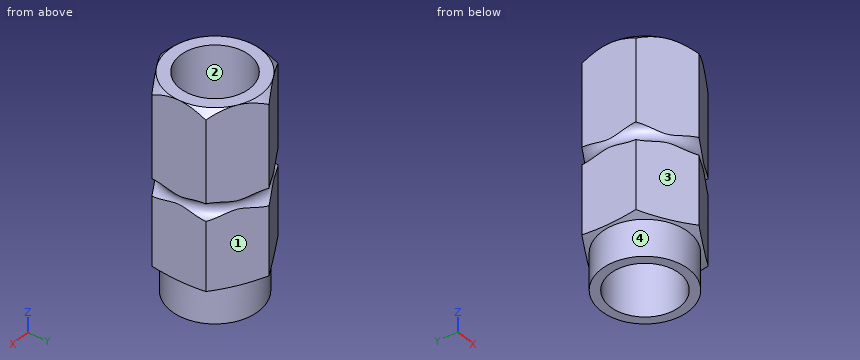
```python
from build123d import *

# Parameters (mm, degrees)
SKETCH1_R      = 9.525
EXTRUDE1_DEPTH = 59
SKETCH2_R      = 2.38125


with BuildPart() as part:
    # Sketch1 → Extrude1 (new body)
    with BuildSketch(Plane.XY):
        Polygon((-12.7, 7.332348419), (-12.7, -7.332348419), (0, -14.664696837), (12.7, -7.332348419), (12.7, 7.332348419), (0, 14.664696837), align=None)
        Circle(SKETCH1_R, mode=Mode.SUBTRACT)
    extrude(amount=-EXTRUDE1_DEPTH)

    # Sketch2 → Cut-Revolve3 (revolve, cut)
    with BuildSketch(Plane(origin=(0, 0, 0), x_dir=(0, 0, -1), z_dir=(1, 0, 0)), mode=Mode.PRIVATE) as cut_revolve3_sk:
        Polygon((59, 14.664696837), (48.285996634, 14.664696837), (49, 12), (59, 12), align=None)
        Polygon((1.964696837, 14.664696837), (0, 14.664696837), (0, 12.7), align=None)
        with Locations((26.9875, 14.78125)):
            Circle(SKETCH2_R)
    revolve(cut_revolve3_sk.sketch.rotate(Axis((0, 0, 0), (0, 0, -1)), 90), axis=Axis((0, 0, 0), (0, 0, -1)), mode=Mode.SUBTRACT)


solid = part.part
```
For this review, take the finished solid that the model builds, in its own axes (mm). Face numbers are marked on the shaded views. Round coordinates to 2 decimals unless told otherwise and drop trailing zeros. Write each loop counter-clockwise with the first axis right and the second up, starting at its lowest first coordinate (ties: lowest second). Pieces come first, ordered by that corner, then holes.
1) For line 1 along Y through (x, z) = (0, -39) (3 decimals); line 2 along Y through (x, z) = (4.5, -19); line 3 along X through (y, z) = (-7.75, -36), list the stretches that pass through material, from the lowest coordinate up.
Answer below:
line 1: y = -14.665 to -9.525, 9.525 to 14.665
line 2: y = -12.07 to -8.39, 8.39 to 12.07
line 3: x = -11.98 to -5.54, 5.54 to 11.98
2) Take a section at A-A on z = -15. Give the boundary of the cut face in (x, y) (3 decimals).
Answer below:
outline: (-12.7, -7.332) - (0, -14.665) - (12.7, -7.332) - (12.7, 7.332) - (0, 14.665) - (-12.7, 7.332) - close; hole circle Ø19.05 at (0, 0)
3) Mouldability with a two-part tool opening along X and no side actions: class the marked faces 1, 2, 3 and 4 as +X half, -X half, draft (parallel to the pull), parting line (faces both ways), or undercut.
Answer below:
face 1: +X half
face 2: undercut
face 3: -X half
face 4: parting line
4) Insertion check: pin 1 Ø15 at (x, y) = (0, 0) entering from +Z. The pin has a flat end and moves straight along its axis. Give the tip position at first contact, or say it passes through.
Answer below:
pin 1: passes through
